```python
from build123d import *

# Parameters (mm, degrees)
SKETCH1_W           = 25.4
SKETCH1_H           = 12.7
BOSS_EXTRUDE1_DEPTH = 1.5875


with BuildPart() as part:
    # Sketch1 → Boss-Extrude1 (new body)
    with BuildSketch(Plane(origin=(0, 0, 0), x_dir=(1, 0, 0), z_dir=(0, 1, 0))):
        Polygon((-44.45, -95.25), (44.45, -95.25), (44.45, -82.55), (44.45, 95.25), (-44.45, 95.25), align=None)
        with Locations((57.15, -88.9)):
            Rectangle(SKETCH1_W, SKETCH1_H)
    extrude(amount=BOSS_EXTRUDE1_DEPTH)


solid = part.part
```
Source: CAD feature listing. Evaluate the final solid. Frame: model axes, mm. Give positions to 0.01 mm unless a question says otherwise; leave off trailing zeros. Loops run counter-clockwise (first coordinate to the right, second up) from the corner with the lowest first, then second, coordinate; pieces in that order, holes last. Notation, with made-up numbers: (63.5, 47) -> (68.5, 47) arc R16 cw to (68.5, 78) -> close; hole circle Ø2 at (16, -29.5). An arc over 180 degrees is marked (long way). Use a Markdown table: item, result. Add a question column.
(1) Ray query, line 1 (X direction, y = 0.25, z = -39.5); line 2 (Z direction, x = 59, y = 0.2). Return the intervals inside material, ascending.
(2) Section query C-C (z = -53.5). Output: boundary loops of the cut face in (x, y), then the cut area to 3 significant figures.
(3) First-contact query: pin 1 Ø0.5 at (y, z) = (1, -22.5) entering from +X. Flat tip, straight axial feed; report the tip coordinate or a pass-through.
(4) Section query A-A (y = 1.3). Output: boundary loops of the cut face in (x, z), then the cut area to 3 significant figures.
(5) Section query B-B (x = 55). Output: boundary loops of the cut face in (y, z).
Checked values:
| question | item | result |
|---|---|---|
| 1 | line 1 | -44.45 to 44.45 |
| 1 | line 2 | 82.55 to 95.25 |
| 2 | outline | (-44.45, 0) -> (44.45, 0) -> (44.45, 1.59) -> (-44.45, 1.59) -> close |
| 2 | area | 141 mm^2 |
| 3 | pin 1 | x = 44.45 |
| 4 | outline | (-44.45, -95.25) -> (44.45, -95.25) -> (44.45, 82.55) -> (69.85, 82.55) -> (69.85, 95.25) -> (-44.45, 95.25) -> close |
| 4 | area | 17,300 mm^2 |
| 5 | outline | (0, 82.55) -> (1.59, 82.55) -> (1.59, 95.25) -> (0, 95.25) -> close |
